Work out the finished part from the listing and answer in its coordinate system (mm). A direction names the side the tool comes from. Coordinates: 2 decimals unless noted, no trailing zeros. Write each loop counter-clockwise with the first axis right and the second up, starting at its lowest first coordinate (ties: lowest second). Pieces come first, ordered by that corner, then holes. Notation, with made-up numbers: M -20.75,68 L -16.75,68 A38 ccw -16.75,106 Z; hole C 78,48.5 d8. An arc over 180 degrees is marked long. Use CSV: the item, a comma, the result in double quotes.
from build123d import *

# Parameters (mm, degrees)
F1_DEPTH = 63.5
F0_W     = 16.735083
F0_H     = 4.7498
F2_DEPTH = 25.4
F3_DEPTH = 7.9375
F5_R     = 6.35


with BuildPart() as f1:
    # F0 (on Front) → F1 (new body, symmetric)
    with BuildSketch(Plane.XZ):
        Polygon((41.275, -9.525), (41.275, 9.525), (22.225, 9.525), (-41.275, 9.525), (-41.275, -9.525), align=None)
    extrude(amount=F1_DEPTH, both=True)

    # F0 (on Front) → F2 (join, symmetric)
    with BuildSketch(Plane.XZ):
        with Locations((68.692541, 64.3001)):
            Rectangle(F0_W, F0_H)
        with BuildLine():
            Line((22.225, 9.525), (41.275, 9.525))
            Line((41.275, 9.525), (41.275, 27.0002))
            ThreePointArc((41.275, 27.0002), (45.92468, 38.22552), (57.15, 42.8752))
            Line((57.15, 42.8752), (60.325, 42.8752))
            Line((60.325, 42.8752), (60.325, 61.9252))
            Line((60.325, 61.9252), (57.15, 61.9252))
            ThreePointArc((57.15, 61.9252), (32.454296, 51.695904), (22.225, 27.0002))
            Line((22.225, 27.0002), (22.225, 9.525))
        make_face()
    extrude(amount=F2_DEPTH, both=True)

    # F0 (on Front) → F3 (join, symmetric)
    with BuildSketch(Plane.XZ):
        with BuildLine():
            Line((-41.275, 9.525), (22.225, 9.525))
            Line((22.225, 9.525), (22.225, 27.0002))
            ThreePointArc((22.225, 27.0002), (32.454296, 51.695904), (57.15, 61.9252))
            add(Edge.make_bspline(
                [(-41.275, 9.525), (-41.275, 23.724295), (-9.110224, 61.9252), (57.15, 61.9252)],
                knots=[0, 0, 0, 0, 111.504536, 111.504536, 111.504536, 111.504536], degree=3))
        make_face()
    extrude(amount=F3_DEPTH, both=True)

    # F0 (on Front) → F4 (revolve)
    with BuildSketch(Plane.XZ):
        Polygon((77.060083, 61.9252), (77.060083, 42.8752), (77.060083, 38.1), (111.125, 38.1), (111.125, 66.675), (77.060083, 66.675), align=None)
    revolve(axis=Axis((77.060083, 0, 52.3875), (0, 0, 1)))

    # F5
    f5_edges = [f1.edges().sort_by_distance(p)[0] for p in [
        (41.275, -63.5, 0),
        (-41.275, -63.5, 0),
        (-41.275, 63.5, 0),
        (41.275, 63.5, 0),
    ]]
    fillet(f5_edges, radius=F5_R)


solid = f1.part
Item 1: A tool of negligible diameter and unlimited length cuts with its end or side. For faces 1 (the face through (79, 0, 38.1)), 2 (the face through (38, -25.4, 36)), 3 (the face through (1, 7.938, 30)), from which of +Z, -Z, +X, -X, +Y, -Y can it reach the whole face along a straight path? Write none if from no direction.
Answer:
face 1,"-Z, +X, +Y, -Y"
face 2,"+Z, -X, -Y"
face 3,"+Z, -X, +Y"
Item 2: The part is cut by section B-B (x = 79). Write down the section's boundary in (y, z) (3 decimals).
Answer:
outline,"M -34.01,38.1 L 34.01,38.1 L 34.01,66.675 L -34.01,66.675 Z"
Item 3: Consider probe 1 along Y at (x, z) = (43.5, 52.5); probe 2 along X at (y, z) = (13, -1.5) (3 decimals); probe 3 along Y at (x, z) = (6, 25). Determine where each line is inside the solid, lowest interval first.
Answer:
probe 1,"y = -25.4 to 25.4"
probe 2,"x = -41.275 to 41.275"
probe 3,"y = -7.94 to 7.94"
Item 4: The part is cut by section C-C (y = -22). Write down the section's boundary in (x, z) (3 decimals), then the cut area to 3 significant figures.
Answer:
outline,"M -41.275,-9.525 L 41.275,-9.525 L 41.275,27 A15.875 cw 51.052,41.657 L 51.052,38.1 L 103.068,38.1 L 103.068,66.675 L 51.052,66.675 L 51.052,61.389 A34.925 ccw 22.225,27 L 22.225,9.525 L -41.275,9.525 Z"
area,"4,030 mm2"
Item 5: Given pin 1 (1 mm diameter, centred on x = -2.5, y = 24, fed in from +Z) (3 decimals); pin 2 (5 mm diameter, centred on y = 17, z = 17.5, fed in from -X) (3 decimals); pin 3 (10 mm diameter, centred on y = 0, z = 49, fed in from -X), each flat-ended and moving along its own axis, determine where each tip first touches the part or whether it passes through.
Answer:
pin 1,"stops at z = 9.525"
pin 2,"stops at x = 22.225"
pin 3,"stops at x = -12.4"
Item 6: The part is cut by section A-A (y = -47). Write down the section's boundary in (x, z) (3 decimals).
Answer:
outline,"M -41.275,-9.525 L 41.275,-9.525 L 41.275,9.525 L -41.275,9.525 Z"
